The listing builds one solid part. Answer for the finished solid, in the listing's coordinates (mm). A direction names the side the tool comes from. Coordinates: 2 decimals unless noted, no trailing zeros. Loops run counter-clockwise (first coordinate to the right, second up) from the corner with the lowest first, then second, coordinate; pieces in that order, holes last. Notation, with made-up numbers: (79.5, -33.5) - (100.5, -33.5) arc R20 ccw to (100.5, -18.5) - close; hole circle Ø2 at (85, -10.75). An arc over 180 degrees is marked (long way). Return JSON: item names as keys, results as strings. Group by question number.
1. Section C-C (y = -58) is taken. Write down the section's boundary in (x, z), and give its area (3 significant figures).
2. Section B-B (y = -20) is taken. Write down the section's boundary in (x, z).
3. Section D-D (x = 6) is taken. Write down the section's boundary in (y, z), and give its area (3 significant figures).
4. Section A-A (z = 0.7) is taken. Write down the section's boundary in (x, y), and give its area (3 significant figures).
5. Find the intervals of material crossed by line 1 along X through (y, z) = (-29, 0.25); line 2 along X through (y, z) = (-20.5, 2.2); line 3 along X through (y, z) = (-57.5, 2.75), in increasing order.
6. The mould has two halves that part along Y. Classify faces 1 (the face through (43, -45, 0)), 2 (the face through (42.62, -89.83, 1.48)), 3 (the face through (98.71, -19.93, 1.52)): pulls with the +Y half, pulls with the -Y half, needs draft (parallel to the pull), parting line crosses it, or undercut.
7. Each of these flat-tipped pins is pushed along its axis until it touches: P1, Ø1, axis at y = -41.5, z = 1, coming from the +X side; P2, Ø0.9, axis at x = 84.5, z = 2, coming from the +Y side. Where does it stop, or does it pass through?
8. Which of the six approach directions +Z, -Z, +X, -X, +Y, -Y give full straight-line access (tool end or side, diameter ignored) to faces 4 (the face through (105.208, 1, 2)), 5 (the face through (-10.147, -56.414, 1.479))?
```python
from build123d import *

# Parameters (mm, degrees)
BOSS_EXTRUDE1_DEPTH = 3
SKETCH2_W           = 30
SKETCH2_H           = 3
SKETCH2_R           = 1.5
CUT_EXTRUDE1_DEPTH  = 3
SKETCH3_R           = 1.6
CUT_EXTRUDE2_DEPTH  = 3


with BuildPart() as part:
    # Sketch1 → Boss-Extrude1 (new body)
    with BuildSketch(Plane.XY):
        Polygon((-33.355339059, 3), (118.208152802, 3), (116.505826096, -94.526231635), (-33.355339059, -85), align=None)
    extrude(amount=BOSS_EXTRUDE1_DEPTH)

    # Sketch2 → Cut-Extrude1 (cut)
    with BuildSketch(Plane.XY.offset(3)):
        with Locations((90.208152802, 1.5)):
            Rectangle(SKETCH2_W, SKETCH2_H)
        with Locations((80.208152802, -20)):
            Circle(SKETCH2_R)
        with Locations((100.208152802, -20)):
            Circle(SKETCH2_R)
    extrude(amount=-CUT_EXTRUDE1_DEPTH, mode=Mode.SUBTRACT)

    # Sketch3 → Cut-Extrude2 (cut)
    with BuildSketch(Plane(origin=(0, 0, 0), x_dir=(-1, 0, 0), z_dir=(0, 0, -1))):
        with Locations((10.355339059, -28)):
            Circle(SKETCH3_R)
        with Locations((10.355339059, -58)):
            Circle(SKETCH3_R)
    extrude(amount=-CUT_EXTRUDE2_DEPTH, mode=Mode.SUBTRACT)


solid = part.part
```
The answers:
{
 "1": {"outline": "(-33.36, 0) - (-11.96, 0) - (-11.96, 3) - (-33.36, 3) - close; (-8.76, 0) - (117.14, 0) - (117.14, 3) - (-8.76, 3) - close", "area": "442 mm2"},
 "2": {"outline": "(-33.36, 0) - (78.71, 0) - (78.71, 3) - (-33.36, 3) - close; (81.71, 0) - (98.71, 0) - (98.71, 3) - (81.71, 3) - close; (101.71, 0) - (117.81, 0) - (117.81, 3) - (101.71, 3) - close"},
 "3": {"outline": "(-87.5, 0) - (3, 0) - (3, 3) - (-87.5, 3) - close", "area": "272 mm2"},
 "4": {"outline": "(-33.36, -85) - (116.51, -94.53) - (118.21, 3) - (105.21, 3) - (105.21, 0) - (75.21, 0) - (75.21, 3) - (-33.36, 3) - close; hole circle Ø3.2 at (-10.36, -58); hole circle Ø3.2 at (-10.36, -28); hole circle Ø3 at (80.21, -20); hole circle Ø3 at (100.21, -20)", "area": "13,900 mm2"},
 "5": {"line 1": "x = -33.36 to -11.6, -9.11 to 117.65", "line 2": "x = -33.36 to 78.79, 81.62 to 98.79, 101.62 to 117.8", "line 3": "x = -33.36 to -11.88, -8.84 to 117.15"},
 "6": {"face 1": "needs draft", "face 2": "pulls with the -Y half", "face 3": "undercut"},
 "7": {"P1": "stops at x = 117.44", "P2": "stops at y = 0"},
 "8": {"face 4": "+Z, -Z, +Y", "face 5": "+Z, -Z"}
}
